Input: part model. Units: mm. Frame: model coordinates. A direction names the side the tool comes from. Round coordinates to 2 decimals unless told otherwise and drop trailing zeros. Order: outer loops, then holes, each group sorted by start corner. A loop starts at its lowest first (then second) coordinate and runs counter-clockwise, first axis right, second up. Notation, with made-up numbers: (-36, -30.5) - (7, -30.5) arc R18 ccw to (7, 2.5) - close; hole circle Ø3 at (58.25, -27.5). An arc over 180 degrees is marked (long way). One line per item, written item: value. Start each with the question number.
from build123d import *

# Parameters (mm, degrees)
BOSS_EXTRUDE1_DEPTH = 3.5
SKETCH2_R           = 0.9
BOSS_EXTRUDE2_DEPTH = 1.6
CHAMFER1_SIZE       = 0.2
SKETCH3_R           = 3.55
BOSS_EXTRUDE3_DEPTH = 0.8
SKETCH4_W           = 3
SKETCH4_H           = 3
BOSS_EXTRUDE4_DEPTH = 1.2
SKETCH5_W           = 3.8
SKETCH5_H           = 3.8
BOSS_EXTRUDE5_DEPTH = 1.8
SKETCH6_R           = 0.9
CUT_EXTRUDE1_DEPTH  = 2


with BuildPart() as part:
    # Sketch1 → Boss-Extrude1 (new body)
    with BuildSketch(Plane(origin=(0, 0, 0), x_dir=(1, 0, 0), z_dir=(0, 1, 0))):
        Polygon((-6, 5), (-5, 6), (5, 6), (6, 5), (6, -5), (5, -6), (-5, -6), (-6, -5), align=None)
    extrude(amount=BOSS_EXTRUDE1_DEPTH)

    # Sketch2 → Boss-Extrude2 (add)
    with BuildSketch(Plane.XZ):
        with Locations((0, -4.5)):
            Circle(SKETCH2_R)
        with Locations((0, 4.5)):
            Circle(SKETCH2_R)
    extrude(amount=BOSS_EXTRUDE2_DEPTH)

    # Chamfer1
    chamfer1_edges = [part.edges().sort_by_distance(p)[0] for p in [
        (-0.9, -1.6, -4.5),
        (-0.9, -1.6, 4.5),
    ]]
    chamfer(chamfer1_edges, length=CHAMFER1_SIZE)

    # Sketch3 → Boss-Extrude3 (add)
    with BuildSketch(Plane(origin=(0, 3.5, 0), x_dir=(1, 0, 0), z_dir=(0, 1, 0))):
        Circle(SKETCH3_R)
    extrude(amount=BOSS_EXTRUDE3_DEPTH)

    # Sketch4 → Boss-Extrude4 (add)
    with BuildSketch(Plane(origin=(0, 4.3, 0), x_dir=(1, 0, 0), z_dir=(0, 1, 0))):
        Rectangle(SKETCH4_W, SKETCH4_H)
    extrude(amount=BOSS_EXTRUDE4_DEPTH)

    # Sketch5 → Boss-Extrude5 (add)
    with BuildSketch(Plane(origin=(0, 5.5, 0), x_dir=(1, 0, 0), z_dir=(0, 1, 0))):
        Rectangle(SKETCH5_W, SKETCH5_H)
    extrude(amount=BOSS_EXTRUDE5_DEPTH)

    # Sketch6 → Cut-Extrude1 (cut)
    with BuildSketch(Plane(origin=(0, 7.3, 0), x_dir=(1, 0, 0), z_dir=(0, 1, 0))):
        Circle(SKETCH6_R)
    extrude(amount=-CUT_EXTRUDE1_DEPTH, mode=Mode.SUBTRACT)


solid = part.part
Item 1: First-contact query: pin 1 Ø0.5 at (y, z) = (6, 0) entering from +X; pin 2 Ø0.6 at (x, y) = (0, 5) entering from +Z; pin 3 Ø0.5 at (y, z) = (6.5, 0) entering from -X. Flat tips, straight axial feed; report the tip coordinate or a pass-through.
Item 2: Section query B-B on y = 6.75. Return loops of the section in (x, z), and give its area (3 significant figures).
Item 3: Line query: L1, parallel to Z at x = 0, y = 6.6; L2, parallel to Y at x = 2.25, z = -4.5. Output: solid intervals per line, ascending.
Item 4: Reachability of faces 5 (the face through (2, 4.3, 0)), 6 (the face through (-1.9, 6, 0)), 7 (the face through (-0.195, -0.69, -5.379)) from +Z, -Z, +X, -X, +Y, -Y: full face, straight path, thin tool, end or side. Return the list, or none.
Item 5: Pull-direction query (Y, two-part tool) for faces 1 (the face through (0, 0, 0)), 2 (the face through (-5.5, 1.7, 5.5)), 3 (the face through (0, 5, 1.5)), 4 (the face through (1.5, 5, 0)); classes: released by +Y, released by -Y, zero draft, split by the parting line, or undercut.
Item 6: Section query A-A on z = 0. Return loops of the section in (x, y).
Item 7: Section query D-D on x = 2.25. Return loops of the section in (y, z), and give its area (3 significant figures).
Geometry results:
1. pin 1: stops at x = 1.9
1. pin 2: stops at z = 1.5
1. pin 3: stops at x = -1.9
2. outline: (-1.9, -1.9) - (1.9, -1.9) - (1.9, 1.9) - (-1.9, 1.9) - close; hole circle Ø1.8 at (0, 0)
2. area: 11.9 mm^2
3. L1: z = -1.9 to -0.9, 0.9 to 1.9
3. L2: y = 0 to 3.5
4. face 5: none
4. face 6: +Z, -Z, -X, +Y
4. face 7: -Y
5. face 1: released by -Y
5. face 2: zero draft
5. face 3: undercut
5. face 4: undercut
6. outline: (-6, 0) - (6, 0) - (6, 3.5) - (3.55, 3.5) - (3.55, 4.3) - (1.5, 4.3) - (1.5, 5.5) - (1.9, 5.5) - (1.9, 7.3) - (0.9, 7.3) - (0.9, 5.3) - (-0.9, 5.3) - (-0.9, 7.3) - (-1.9, 7.3) - (-1.9, 5.5) - (-1.5, 5.5) - (-1.5, 4.3) - (-3.55, 4.3) - (-3.55, 3.5) - (-6, 3.5) - close
7. outline: (0, -6) - (3.5, -6) - (3.5, -2.75) - (4.3, -2.75) - (4.3, 2.75) - (3.5, 2.75) - (3.5, 6) - (0, 6) - close
7. area: 46.4 mm^2
